CAD build for the part. Positions are in the model's coordinates, mm. Face numbers are marked on the shaded views. A direction names the side the tool comes from. Round coordinates to 2 decimals unless told otherwise and drop trailing zeros. Loops run counter-clockwise (first coordinate to the right, second up) from the corner with the lowest first, then second, coordinate; pieces in that order, holes last. Notation, with made-up numbers: M 6.25,18.25 L 26.25,18.25 A22 ccw 26.25,51.25 Z; hole C 24,73.25 d1. An arc over 180 degrees is marked long. Use a Markdown table: item, result. Add a question column.
(1) Which spindle directions (+Z, -Z, +X, -X, +Y, -Y) get a long thin tool onto all of the face, cutting with end or side? Do the marked faces 1, 2 and 3. Say none if no direction does.
(2) Band-saw the part on A-A, the plane y = 0. Write the cut outline in (x, z), and give its area (3 significant figures).
(3) Two-plate mould, pull along X, no slides. Class the marked faces 4, 5 and 6: released by +X, released by -X, zero draft, split by the parting line, or undercut.
(4) Band-saw the part on B-B, the plane x = 29.5. Write the cut outline in (y, z), and give its area (3 significant figures).
(5) Band-saw the part on C-C, the plane z = 0. Write the cut outline in (x, y).
(6) Wall check: L1, parallel to Y at x = 5, z = 20; L2, parallel to X at y = -12, z = 0; L3, parallel to Y at x = 10.85, z = -1. Give the ranges that are in metal, low to high.
(7) Flat gauge pins, fed straight in: P1, Ø3, axis at x = 28, y = 8.5, coming from the -Z side; P2, Ø4, axis at y = 2, z = -12, coming from the +X side; P3, Ø6, axis at y = 9.5, z = -21, coming from the +X side. Where does each tip first touch, or does it go through?
from build123d import *

# Parameters (mm, degrees)
SKETCH1_R               = 4.7625
BOSS_EXTRUDE1_DEPTH     = 50
CUT_EXTRUDE3_DEPTH      = 17
CUT_EXTRUDE3_DEPTH_BACK = 17
SKETCH5_R               = 4.7625
CUT_EXTRUDE2_DEPTH      = 17
CUT_EXTRUDE2_DEPTH_BACK = 17
CUT_EXTRUDE4_DEPTH      = 37
CUT_EXTRUDE4_DEPTH_BACK = 37


with BuildPart() as part:
    # Sketch1 → Boss-Extrude1 (new body)
    with BuildSketch(Plane(origin=(0, 0, 0), x_dir=(0, 0, -1), z_dir=(1, 0, 0))):
        with BuildLine():
            Line((-20, 16), (0, 16))
            Line((0, 16), (20, 16))
            ThreePointArc((20, 16), (36, 0), (20, -16))
            Line((20, -16), (0, -16))
            Line((0, -16), (-20, -16))
            ThreePointArc((-20, -16), (-36, 0), (-20, 16))
        make_face()
        with Locations((-20, 0)):
            Circle(SKETCH1_R, mode=Mode.SUBTRACT)
        with Locations((20, 0)):
            Circle(SKETCH1_R, mode=Mode.SUBTRACT)
    extrude(amount=BOSS_EXTRUDE1_DEPTH)

    # Sketch3 → Cut-Extrude3 (cut, two sides)
    with BuildSketch(Plane(origin=(0, 0, 0), x_dir=(1, 0, 0), z_dir=(0, 1, 0))) as cut_extrude3_sk:
        with BuildLine():
            Line((6, 36), (30.35, 11.65))
            ThreePointArc((30.35, 11.65), (35.175588002, 0), (30.35, -11.65))
            Line((30.35, -11.65), (6, -36))
            Line((6, -36), (6, -40.720576269))
            Line((6, -40.720576269), (53.537884165, -40.720576269))
            Line((53.537884165, -40.720576269), (53.537884165, 49.648939658))
            Line((53.537884165, 49.648939658), (6, 49.648939658))
            Line((6, 49.648939658), (6, 36))
        make_face()
    extrude(amount=CUT_EXTRUDE3_DEPTH, mode=Mode.SUBTRACT)
    extrude(cut_extrude3_sk.sketch, amount=-CUT_EXTRUDE3_DEPTH_BACK, mode=Mode.SUBTRACT)

    # Sketch5 → Cut-Extrude2 (cut, two sides)
    with BuildSketch(Plane(origin=(0, 0, 0), x_dir=(1, 0, 0), z_dir=(0, 1, 0))) as cut_extrude2_sk:
        with Locations((18.7, 0)):
            Circle(SKETCH5_R)
    extrude(amount=CUT_EXTRUDE2_DEPTH, mode=Mode.SUBTRACT)
    extrude(cut_extrude2_sk.sketch, amount=-CUT_EXTRUDE2_DEPTH_BACK, mode=Mode.SUBTRACT)

    # Sketch7 → Cut-Extrude4 (cut, two sides)
    with BuildSketch(Plane.XY) as cut_extrude4_sk:
        with BuildLine():
            Line((56.351176003, -7.14375), (14, -7.14375))
            ThreePointArc((14, -7.14375), (6.85625, 0), (14, 7.14375))
            Line((14, 7.14375), (56.351176003, 7.14375))
            ThreePointArc((56.351176003, 7.14375), (63.494926003, 0), (56.351176003, -7.14375))
        make_face()
    extrude(amount=CUT_EXTRUDE4_DEPTH, mode=Mode.SUBTRACT)
    extrude(cut_extrude4_sk.sketch, amount=-CUT_EXTRUDE4_DEPTH_BACK, mode=Mode.SUBTRACT)

    # Sketch10 → Cut-Revolve1 (revolve, cut)
    with BuildSketch(Plane(origin=(0, 0, 0), x_dir=(1, 0, 0), z_dir=(0, 1, 0))):
        with BuildLine():
            Line((3.7, 4), (3.7, -4))
            ThreePointArc((3.7, -4), (5.794186515, -9.055813485), (10.85, -11.15))
            Line((10.85, -11.15), (10.85, 11.15))
            ThreePointArc((10.85, 11.15), (5.794186515, 9.055813485), (3.7, 4))
        make_face()
    revolve(axis=Axis((10.85, 0, -11.15), (0, 0, 1)), mode=Mode.SUBTRACT)


solid = part.part
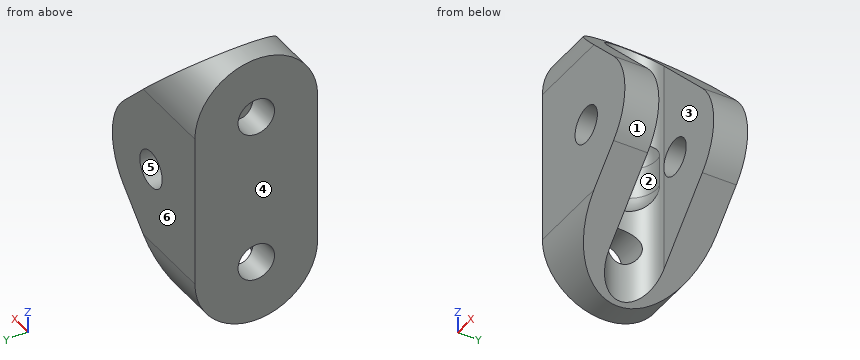
Return value:
| question | item | result |
|---|---|---|
| 1 | face 1 | +X, +Y, -Y |
| 1 | face 2 | none |
| 1 | face 3 | +Z, -Z, +X |
| 2 | outline | M 0,-36 L 6,-36 L 6.86,-35.14 L 6.86,-24.76 L 0,-24.76 Z; M 0,-15.24 L 6.86,-15.24 L 6.86,-9.93 A7.15 cw 3.7,-4 L 3.7,4 A7.15 cw 6.86,9.93 L 6.86,15.24 L 0,15.24 Z; M 0,24.76 L 6.86,24.76 L 6.86,35.14 L 6,36 L 0,36 Z |
| 2 | area | 311 mm^2 |
| 3 | face 4 | released by -X |
| 3 | face 5 | undercut |
| 3 | face 6 | zero draft |
| 4 | outline | M -16,-12.5 L -7.14,-12.5 L -7.14,12.5 L -16,12.5 Z; M 7.14,-12.5 L 16,-12.5 L 16,12.5 L 7.14,12.5 Z |
| 4 | area | 443 mm^2 |
| 5 | outline | M 0,-16 L 13.94,-16 L 13.94,-7.14 A7.14 cw 12.44,-6.97 A7.15 cw long 12.44,6.97 A7.14 cw 13.94,7.14 L 13.94,16 L 0,16 Z; M 23.46,-16 L 35.18,-16 L 35.18,-7.14 L 23.46,-7.14 Z; M 23.46,7.14 L 35.18,7.14 L 35.18,16 L 23.46,16 Z |
| 6 | L1 | -16 to -4.76, 4.76 to 16 |
| 6 | L2 | 0 to 13.94, 23.46 to 35.18 |
| 6 | L3 | -16 to -7.15, 7.15 to 16 |
| 7 | P1 | z = -15.5 |
| 7 | P2 | x = 8.08 |
| 7 | P3 | x = 24 |
